from build123d import *

# Parameters (mm, degrees)
SKETCH1_W                 = 43.18
SKETCH1_H                 = 25.4
BASE_DEPTH                = 37.592
SKETCH2_W                 = 12.065
SKETCH2_H                 = 11.938
LINACTSLOT_DEPTH          = 51.24387091
MOUTINGHOLES_D            = 2.7051
MOUTINGHOLES_DEPTH        = 14.478
MOUTINGHOLES_TIP          = 0.81269403
MOTORSLOT_DEPTH           = 51.24387091
MOTORMOUNTINGHOLES2_D     = 2.2606
MOTORMOUNTINGHOLES2_DEPTH = 11.43
MOTORMOUNTINGHOLES2_TIP   = 0.679152758
F_8_32_TAPPED_HOLE1_D     = 3.4544
F_8_32_TAPPED_HOLE1_DEPTH = 7.62
F_8_32_TAPPED_HOLE1_TIP   = 1.037806461
SKETCH23_W                = 43.18
SKETCH23_H                = 15.24
CUT_EXTRUDE1_DEPTH        = 2.032


with BuildPart() as part:
    # Sketch1 → Base (new body)
    with BuildSketch(Plane(origin=(0, 0, 0), x_dir=(1, 0, 0), z_dir=(0, 1, 0))):
        Rectangle(SKETCH1_W, SKETCH1_H)
    extrude(amount=BASE_DEPTH)

    # Sketch2 → LinActSlot (cut, through all)
    with BuildSketch(Plane.XY.offset(12.7)):
        with Locations((0, 31.623)):
            Rectangle(SKETCH2_W, SKETCH2_H)
    extrude(amount=-LINACTSLOT_DEPTH, mode=Mode.SUBTRACT)

    # MoutingHoles
    with Locations(Plane(origin=(14.160350453, 37.592, 8.373414988), x_dir=(-1, 0, 0), z_dir=(0, 1, 0))):
        with Locations((1.460350453, -4.563414988), (26.860350453, -4.563414988)):
            Hole(MOUTINGHOLES_D / 2, depth=MOUTINGHOLES_DEPTH)
            with Locations((0, 0, -(MOUTINGHOLES_DEPTH + MOUTINGHOLES_TIP / 2))):  # 118° drill point
                Cone(0, MOUTINGHOLES_D / 2, MOUTINGHOLES_TIP, mode=Mode.SUBTRACT)

    # Sketch11 → MotorSlot (cut, through all)
    with BuildSketch(Plane(origin=(0, 0, -12.7), x_dir=(-1, 0, 0), z_dir=(0, 0, -1))):
        with BuildLine():
            Line((15.875, 5.08), (15.875, 5.715))
            ThreePointArc((15.875, 5.715), (13.085192091, 12.450192091), (6.35, 15.24))
            Line((6.35, 15.24), (5.08, 15.24))
            ThreePointArc((5.08, 15.24), (-1.655192091, 12.450192091), (-4.445, 5.715))
            Line((-4.445, 5.715), (-4.445, 5.08))
            Line((-4.445, 5.08), (-4.445, 0))
            Line((-4.445, 0), (15.875, 0))
            Line((15.875, 0), (15.875, 5.08))
        make_face()
    extrude(amount=-MOTORSLOT_DEPTH, mode=Mode.SUBTRACT)

    # MotorMountingHoles2
    with Locations(Plane(origin=(0, 0, -12.7), x_dir=(-1, 0, 0), z_dir=(0, 0, -1))):
        with Locations((18.215, 5.715), (-6.785, 5.715)):
            Hole(MOTORMOUNTINGHOLES2_D / 2, depth=MOTORMOUNTINGHOLES2_DEPTH)
            with Locations((0, 0, -(MOTORMOUNTINGHOLES2_DEPTH + MOTORMOUNTINGHOLES2_TIP / 2))):  # 118° drill point
                Cone(0, MOTORMOUNTINGHOLES2_D / 2, MOTORMOUNTINGHOLES2_TIP, mode=Mode.SUBTRACT)

    # #8-32 Tapped Hole1
    with Locations(Plane.XY.offset(12.7)):
        with Locations((-14.605, 25.146), (14.605, 25.146)):
            Hole(F_8_32_TAPPED_HOLE1_D / 2, depth=F_8_32_TAPPED_HOLE1_DEPTH)
            with Locations((0, 0, -(F_8_32_TAPPED_HOLE1_DEPTH + F_8_32_TAPPED_HOLE1_TIP / 2))):  # 118° drill point
                Cone(0, F_8_32_TAPPED_HOLE1_D / 2, F_8_32_TAPPED_HOLE1_TIP, mode=Mode.SUBTRACT)

    # Sketch23 → Cut-Extrude1 (cut)
    with BuildSketch(Plane(origin=(0, 0, -12.7), x_dir=(-1, 0, 0), z_dir=(0, 0, -1))):
        with Locations((0, 7.62)):
            Rectangle(SKETCH23_W, SKETCH23_H)
    extrude(amount=-CUT_EXTRUDE1_DEPTH, mode=Mode.SUBTRACT)


solid = part.part
Design review of the part built by this model. Coordinates are the model's own, in mm. A direction names the side the tool comes from. Round coordinates to 2 decimals unless told otherwise and drop trailing zeros. Order: outer loops, then holes, each group sorted by start corner. A loop starts at its lowest first (then second) coordinate and runs counter-clockwise, first axis right, second up.
1) Consider section D-D (x = 9). State the section outline as (y, z) points.
The answers:
outline: (0, -10.67) - (15.24, -10.67) - (15.24, -12.7) - (37.59, -12.7) - (37.59, 12.7) - (0, 12.7) - close
2) Consider section B-B (z = -5.5). Count the separate pieces of the cut face and the enclosed holes in it, plus the area to 3 significant figures.
The answers:
separate pieces: 1
enclosed holes: 2
area: 1,200 mm2
3) Machinability: for faces 5 (the flat face through (6.032, 32, 0)), 6 (the cylindrical face through (16.33, 25.22, 8.84)), 7 (the cylindrical face through (5.952, 6.479, -5.903)), 8 (the cylindrical face through (1.581, 12.524, 0.852)), which of the approach directions +Z, -Z, +X, -X, +Y, -Y give a long, thin tool a straight path to every point of the face, cutting with its end or side? Answer none if there is none.
The answers:
face 5: +Z, -Z, +Y
face 6: +Z
face 7: -Z
face 8: +Z, -Z, -Y
4) For L1, parallel to X at y = 34.25, z = 3.81; L2, parallel to X at y = 30.5, z = -1.75; L3, parallel to X at y = 4.5, z = -4 (3 decimals), list the stretches that pass through material, from the lowest coordinate up.
The answers:
L1: x = -21.59 to -14.05, -11.35 to -6.03, 6.03 to 11.35, 14.05 to 21.59
L2: x = -21.59 to -6.03, 6.03 to 21.59
L3: x = -21.59 to -15.875, 4.445 to 21.59
5) Clearance check with flat-ended pins moving along their axes: pin 1 Ø1.6 at (x, z) = (12.7, 3.81) entering from +Y; pin 2 Ø6 at (x, y) = (0, 28) entering from -Z; pin 3 Ø17 at (x, y) = (2.5, 5.5) entering from -Z; pin 4 Ø1.4 at (x, y) = (-18.215, 5.715) entering from -Z. State where each tip first meets the part, or that it passes through.
The answers:
pin 1: stops at y = 22.78
pin 2: stops at z = -12.7
pin 3: stops at z = -10.67
pin 4: stops at z = -1.01
6) Draft analysis for pull direction Z (two halves, no side actions). For faces 1 (the conical face through (14.891, 25.236, 4.222)), 2 (the conical face through (12.483, 22.442, 3.72)), 3 (the flat face through (4.445, 3, 1)), 4 (the flat face through (0, 24, -12.7)), state which applies: released by +Z, released by -Z, zero draft, split by the parting line, or undercut.
The answers:
face 1: released by +Z
face 2: undercut
face 3: zero draft
face 4: released by -Z
7) Consider section C-C (y = 11). State the section outline as (x, z) points, plus the area to 3 significant figures.
The answers:
outline: (-21.59, -10.67) - (-14.27, -10.67) - (-14.27, 12.7) - (-21.59, 12.7) - close; (2.84, -10.67) - (21.59, -10.67) - (21.59, 12.7) - (2.84, 12.7) - close
area: 609 mm2
8) Consider section A-A (y = 32). State the section outline as (x, z) points.
The answers:
outline: (-21.59, -12.7) - (-6.03, -12.7) - (-6.03, 12.7) - (-21.59, 12.7) - close; (6.03, -12.7) - (21.59, -12.7) - (21.59, 12.7) - (6.03, 12.7) - close; hole circle Ø2.71 at (-12.7, 3.81); hole circle Ø2.71 at (12.7, 3.81)
